Can you work these out from the model? Positions are in its coordinate system, mm. A direction names the side the tool comes from. Coordinates: 2 decimals unless noted, no trailing zeros. Loops run counter-clockwise (first coordinate to the right, second up) from the corner with the lowest first, then second, coordinate; pieces in that order, holes last.
```python
from build123d import *

# Parameters (mm, degrees)
SKETCH1_W           = 127
SKETCH1_H           = 190.5
BOSS_EXTRUDE1_DEPTH = 2.54
SKETCH3_W           = 2.54
SKETCH3_H           = 185.42
SKETCH3_W_2         = 116.84
SKETCH3_H_2         = 2.54
BOSS_EXTRUDE2_DEPTH = 19.05
SKETCH4_W           = 2.54
SKETCH4_H           = 15.24
SKETCH4_W_2         = 116.84
SKETCH4_H_2         = 2.54
BOSS_EXTRUDE3_DEPTH = 50.8
FILLET2_R           = 2.54


with BuildPart() as part:
    # Sketch1 → Boss-Extrude1 (new body)
    with BuildSketch(Plane.XY):
        with Locations((63.5, 95.25)):
            Rectangle(SKETCH1_W, SKETCH1_H)
    extrude(amount=BOSS_EXTRUDE1_DEPTH)

    # Sketch3 → Boss-Extrude2 (add)
    with BuildSketch(Plane.XY.offset(2.54)):
        with Locations((1.27, 92.71)):
            Rectangle(SKETCH3_W, SKETCH3_H)
        with Locations((63.5, 189.23)):
            Rectangle(SKETCH3_W_2, SKETCH3_H_2)
        with Locations((125.73, 92.71)):
            Rectangle(SKETCH3_W, SKETCH3_H)
    extrude(amount=BOSS_EXTRUDE2_DEPTH)

    # Sketch4 → Boss-Extrude3 (add)
    with BuildSketch(Plane.XY.offset(21.59)):
        with Locations((1.27, 177.8)):
            Rectangle(SKETCH4_W, SKETCH4_H)
        with Locations((63.5, 189.23)):
            Rectangle(SKETCH4_W_2, SKETCH4_H_2)
        with Locations((125.73, 177.8)):
            Rectangle(SKETCH4_W, SKETCH4_H)
    extrude(amount=BOSS_EXTRUDE3_DEPTH)

    # Fillet2
    fillet2_edges = [part.edges().sort_by_distance(p)[0] for p in [
        (1.27, 170.18, 21.59),
        (0, 190.5, 1.27),
        (125.73, 170.18, 21.59),
        (127, 190.5, 1.27),
    ]]
    fillet(fillet2_edges, radius=FILLET2_R)


solid = part.part
```
Item 1: Suppose I cut it at A-A, the plane z = 64.5. Please give me the cut outline in (x, y).
Results are:
outline: (0, 170.18) - (2.54, 170.18) - (2.54, 185.42) - (0, 185.42) - close; (5.08, 187.96) - (121.92, 187.96) - (121.92, 190.5) - (5.08, 190.5) - close; (124.46, 170.18) - (127, 170.18) - (127, 185.42) - (124.46, 185.42) - close
Item 2: Suppose I cut it at C-C, the plane z = 11. Please give me the cut outline in (x, y).
Results are:
outline: (0, 0) - (2.54, 0) - (2.54, 185.42) - (0, 185.42) - close; (5.08, 187.96) - (121.92, 187.96) - (121.92, 190.5) - (5.08, 190.5) - close; (124.46, 0) - (127, 0) - (127, 185.42) - (124.46, 185.42) - close
Item 3: We'd pull the mould along X, two halves only. Please class faces 1 (the face through (0, 114, 20)), 2 (the face through (49, 0, 2)), 3 (the face through (127, 114, 20)), 4 (the face through (124.46, 112, 21)): +X half, -X half, draft (parallel to the pull), parting line (faces both ways), or undercut.
Results are:
face 1: -X half
face 2: draft
face 3: +X half
face 4: undercut
Item 4: I need wall thicknesses on line 1 along X through (y, z) = (182, 44); line 2 along Z through (x, y) = (85.5, 55.5); line 3 along Y through (x, z) = (113.5, 67.5). Which ranges of each line are inside material? Lowest first, please.
Results are:
line 1: x = 0 to 2.54, 124.46 to 127
line 2: z = 0 to 2.54
line 3: y = 187.96 to 190.5
Item 5: Suppose I cut it at D-D, the plane x = 58. Please give me the cut outline in (y, z).
Results are:
outline: (0, 0) - (190.5, 0) - (190.5, 72.39) - (187.96, 72.39) - (187.96, 2.54) - (0, 2.54) - close
Item 6: On a 3-axis mill with a long thin cutter (end or side, diameter ignored), from which of +Z, -Z, +X, -X, +Y, -Y can I reach the whole of each face in a straight line? I mean faces 5 (the face through (63, 187.96, 37)), 6 (the face through (2.54, 112, 21)), 7 (the face through (63, 97, 0)). Say none if no direction works.
Results are:
face 5: +Z, +X, -X, -Y
face 6: +Z, +Y, -Y
face 7: -Z, +X, -X, +Y, -Y
Item 7: Suppose I cut it at B-B, the plane y = 57. Please give me the cut outline in (x, z).
Results are:
outline: (0, 0) - (127, 0) - (127, 21.59) - (124.46, 21.59) - (124.46, 2.54) - (2.54, 2.54) - (2.54, 21.59) - (0, 21.59) - close
Item 8: I'm going to push flat-ended pins straight in: P1, Ø1, axis at x = 68.5, y = 77.5, coming from the +Z side; P2, Ø0.8, axis at x = 2, y = 62.5, coming from the +Z side; P3, Ø1.5, axis at x = 75.5, z = 20, coming from the -Y side; P4, Ø21, axis at y = 73.5, z = 39, coming from the -X side. Where does each tip first touch, or does it pass through?
Results are:
P1: stops at z = 2.54
P2: stops at z = 21.59
P3: stops at y = 187.96
P4: passes through
